Can you work these out from the model? Positions are in its coordinate system, mm. Coordinates: 2 decimals unless noted, no trailing zeros. Order: outer loops, then holes, each group sorted by start corner. A loop starts at its lowest first (then second) coordinate and runs counter-clockwise, first axis right, second up. Notation, with made-up numbers: M 42,50 L 56,50 A21 ccw 56,88 Z; hole C 8.25,87 d5. An arc over 180 degrees is marked long. Answer as CSV lines item,"result". Start each with the question number.
1. If we section it at A-A (z = 5): Give the number of separate pieces and of enclosed holes in the cut face, plus the area to 3 significant figures.
2. Will these pins go through, and if not, where does the flat tip stop? pin 1 (2 mm diameter, centred on x = 62.5, y = 28, fed in from +Z); pin 2 (1.5 mm diameter, centred on y = 57.5, z = 3.5, fed in from +X); pin 3 (1 mm diameter, centred on y = 48, z = 1, fed in from +X); pin 4 (1.5 mm diameter, centred on x = 129, z = 1.5, fed in from -Y).
3. If we section it at D-D (x = 110): List the corners of the cut face in (y, z) for me, plus the area to 3 significant figures.
4. If we section it at B-B (y = 13): List the corners of the cut face in (x, z) for me.
5. If we section it at C-C (x = 94): List the corners of the cut face in (y, z) for me, plus the area to 3 significant figures.
6. I need wall thicknesses on line 1 along X through (y, z) = (24.5, 4); line 2 along X through (y, z) = (3.5, 2.75); line 3 along X through (y, z) = (10, 4). Which ranges of each line are inside material? Lowest first, please. Write a range as from..to.
```python
from build123d import *

# Parameters (mm, degrees)
ESQUISSE1_W                  = 145
ESQUISSE1_H                  = 40
BOSS_EXTRU_1_DEPTH           = 6
ESQUISSE2_R                  = 1.65
ENL_V_MAT_EXTRU_1_DEPTH      = 1
ENL_V_MAT_EXTRU_1_DEPTH_BACK = 7
ESQUISSE3_W                  = 145
ESQUISSE3_H                  = 30
BOSS_EXTRU_2_DEPTH           = 6
CHANFREIN1_SIZE              = 2
ESQUISSE4_W                  = 57.5
ESQUISSE4_H                  = 54
ENL_V_MAT_EXTRU_2_DEPTH      = 1
ENL_V_MAT_EXTRU_2_DEPTH_BACK = 7
CHANFREIN2_SIZE              = 15
CONG_2_R                     = 5


with BuildPart() as part:
    # Esquisse1 → Boss.-Extru.1 (new body)
    with BuildSketch(Plane.XY):
        with Locations((72.5, 20)):
            Rectangle(ESQUISSE1_W, ESQUISSE1_H)
    extrude(amount=BOSS_EXTRU_1_DEPTH)

    # Esquisse2 → Enlèv. mat.-Extru.1 (cut, two sides)
    with BuildSketch(Plane.XY.offset(6)) as enl_v_mat_extru_1_sk:
        with Locations((62.5, 23)):
            Circle(ESQUISSE2_R)
        with Locations((62.5, 3)):
            Circle(ESQUISSE2_R)
        with Locations((82.5, 3)):
            Circle(ESQUISSE2_R)
        with Locations((82.5, 23)):
            Circle(ESQUISSE2_R)
        with Locations((62.5, 28)):
            Circle(ESQUISSE2_R)
        with Locations((62.5, 8)):
            Circle(ESQUISSE2_R)
        with Locations((82.5, 8)):
            Circle(ESQUISSE2_R)
        with Locations((82.5, 28)):
            Circle(ESQUISSE2_R)
        with Locations((62.5, 33)):
            Circle(ESQUISSE2_R)
        with Locations((62.5, 13)):
            Circle(ESQUISSE2_R)
        with Locations((82.5, 13)):
            Circle(ESQUISSE2_R)
        with Locations((82.5, 33)):
            Circle(ESQUISSE2_R)
    extrude(amount=ENL_V_MAT_EXTRU_1_DEPTH, mode=Mode.SUBTRACT)
    extrude(enl_v_mat_extru_1_sk.sketch, amount=-ENL_V_MAT_EXTRU_1_DEPTH_BACK, mode=Mode.SUBTRACT)

    # Esquisse3 → Boss.-Extru.2 (add)
    with BuildSketch(Plane.XY.offset(6)):
        with Locations((72.5, 55)):
            Rectangle(ESQUISSE3_W, ESQUISSE3_H)
    extrude(amount=-BOSS_EXTRU_2_DEPTH)

    # Chanfrein1
    chanfrein1_edges = [part.edges().sort_by_distance(p)[0] for p in [
        (72.5, 70, 6),
    ]]
    chamfer(chanfrein1_edges, length=CHANFREIN1_SIZE)

    # Esquisse4 → Enlèv. mat.-Extru.2 (cut, two sides)
    with BuildSketch(Plane.XY.offset(6)) as enl_v_mat_extru_2_sk:
        with Locations((28.75, 27)):
            Rectangle(ESQUISSE4_W, ESQUISSE4_H)
        with Locations((116.25, 27)):
            Rectangle(ESQUISSE4_W, ESQUISSE4_H)
    extrude(amount=ENL_V_MAT_EXTRU_2_DEPTH, mode=Mode.SUBTRACT)
    extrude(enl_v_mat_extru_2_sk.sketch, amount=-ENL_V_MAT_EXTRU_2_DEPTH_BACK, mode=Mode.SUBTRACT)

    # Chanfrein2
    chanfrein2_edges = [part.edges().sort_by_distance(p)[0] for p in [
        (87.5, 54, 3),
        (57.5, 54, 3),
    ]]
    chamfer(chanfrein2_edges, length=CHANFREIN2_SIZE)

    # Congé2
    cong_2_edges = [part.edges().sort_by_distance(p)[0] for p in [
        (145, 70, 2),
        (145, 54, 3),
        (102.5, 54, 3),
        (87.5, 39, 3),
        (87.5, 0, 3),
        (57.5, 0, 3),
        (57.5, 39, 3),
        (42.5, 54, 3),
        (0, 54, 3),
        (0, 70, 2),
    ]]
    fillet(cong_2_edges, radius=CONG_2_R)


solid = part.part
```
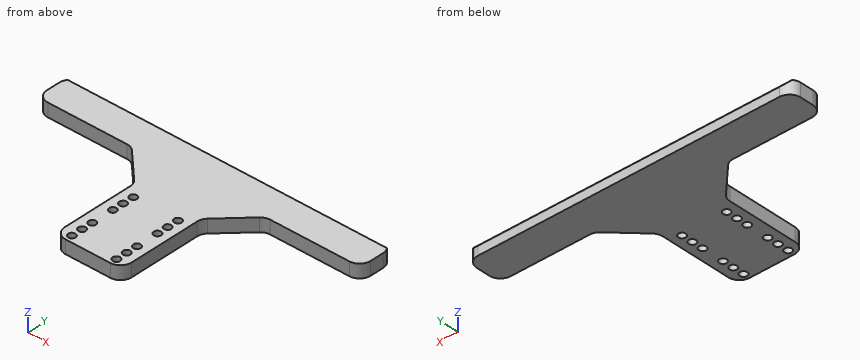
Solved:
1,separate pieces,"1"
1,enclosed holes,"12"
1,area,"3,890 mm²"
2,pin 1,"through"
2,pin 2,"x = 144.94"
2,pin 3,"x = 97"
2,pin 4,"y = 54"
3,outline,"M 54,0 L 70,0 L 70,4 L 68,6 L 54,6 Z"
3,area,"94.0 mm²"
4,outline,"M 57.5,0 L 60.85,0 L 60.85,6 L 57.5,6 Z; M 64.15,0 L 80.85,0 L 80.85,6 L 64.15,6 Z; M 84.15,0 L 87.5,0 L 87.5,6 L 84.15,6 Z"
5,outline,"M 45.5,0 L 70,0 L 70,4 L 68,6 L 45.5,6 Z"
5,area,"145 mm²"
6,line 1,"57.5..61.81, 63.19..81.81, 83.19..87.5"
6,line 2,"57.73..60.93, 64.07..80.93, 84.07..87.27"
6,line 3,"57.5..87.5"
